```python
from build123d import *

# Parameters (mm, degrees)
SKETCH1_W           = 36
SKETCH1_H           = 36
SKETCH1_W_2         = 30
SKETCH1_H_2         = 30
BOSS_EXTRUDE1_DEPTH = 40
SKETCH2_W           = 30
SKETCH2_H           = 30
BOSS_EXTRUDE2_DEPTH = 3
FILLET_1_R          = 2
FILLET_2_R          = 2
FILLET_3_R          = 1


with BuildPart() as part:
    # Sketch1 → Boss-Extrude1 (new body)
    with BuildSketch(Plane(origin=(0, 0, 0), x_dir=(1, 0, 0), z_dir=(0, 1, 0))):
        with Locations((18, 18)):
            Rectangle(SKETCH1_W, SKETCH1_H)
        with Locations((18, 18)):
            Rectangle(SKETCH1_W_2, SKETCH1_H_2, mode=Mode.SUBTRACT)
    extrude(amount=BOSS_EXTRUDE1_DEPTH)

    # Sketch2 → Boss-Extrude2 (add)
    with BuildSketch(Plane.XZ):
        with Locations((18, -18)):
            Rectangle(SKETCH2_W, SKETCH2_H)
    extrude(amount=-BOSS_EXTRUDE2_DEPTH)

    # Скругление1
    fillet_1_edges = [part.edges().sort_by_distance(p)[0] for p in [
        (0, 20, -36),
        (36, 20, -36),
        (36, 20, 0),
        (0, 20, 0),
    ]]
    fillet(fillet_1_edges, radius=FILLET_1_R)

    # Скругление2
    fillet_2_edges = [part.edges().sort_by_distance(p)[0] for p in [
        (0, 0, -18),
        (18, 0, -36),
        (36, 0, -18),
        (18, 0, 0),
        (35.414213562, 0, -0.585786438),
        (35.414213562, 0, -35.414213562),
        (0.585786438, 0, -0.585786438),
        (0.585786438, 0, -35.414213562),
    ]]
    fillet(fillet_2_edges, radius=FILLET_2_R)

    # Скругление3
    fillet_3_edges = [part.edges().sort_by_distance(p)[0] for p in [
        (3, 21.5, -33),
        (3, 21.5, -3),
        (33, 21.5, -3),
        (33, 21.5, -33),
        (3, 40, -18),
        (18, 40, -3),
        (33, 40, -18),
        (18, 40, -33),
        (18, 3, -33),
        (3, 3, -18),
        (18, 3, -3),
        (33, 3, -18),
    ]]
    fillet(fillet_3_edges, radius=FILLET_3_R)


solid = part.part
```
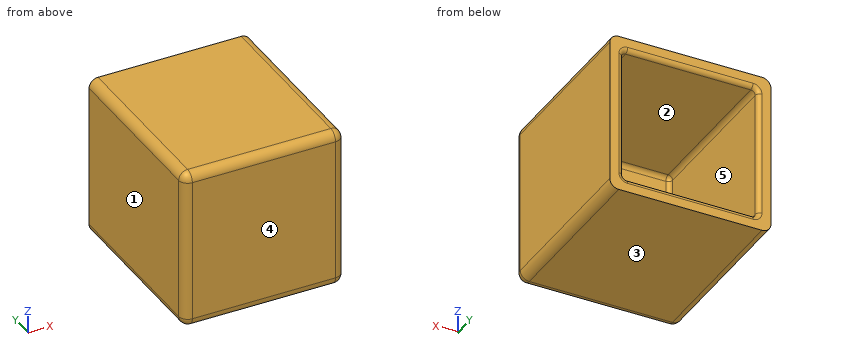
Can you work these out from the model? Positions are in its coordinate system, mm. Face numbers are marked on the shaded views. A direction names the side the tool comes from. Give positions to 0.01 mm unless a question says otherwise; leave off trailing zeros. Order: outer loops, then holes, each group sorted by start corner. A loop starts at its lowest first (then second) coordinate and runs counter-clockwise, first axis right, second up. Notation, with made-up numbers: (17, -17.5) - (31, -17.5) arc R6 ccw to (31, -10.5) - close; hole circle Ø2 at (68.5, -1). An arc over 180 degrees is marked (long way). Use a Markdown table: item, result. Add a question column.
Q1. If we section it at B-B on z = -13.5: Write out the boundary of the cut face in (x, y), plus the area to 3 significant figures.
Q2. On a 3-axis mill with a long thin cutter (end or side, diameter ignored), from which of +Z, -Z, +X, -X, +Y, -Y can I reach the whole of each face in a straight line? I mean the marked faces 4 and 5. Say none if no direction works.
Q3. If we section it at C-C on y = 11: Write out the boundary of the cut face in (x, z), plus the area to 3 significant figures.
Q4. If we section it at A-A on x = 7.5: Write out the boundary of the cut face in (y, z).
Q5. I'm going to push flat-ended pins straight in: pin 1 (8.5 mm diameter, centred on x = 16, z = -14, fed in from +Y); pin 2 (10 mm diameter, centred on x = 22.5, z = -27.5, fed in from +Y). Where does each tip first touch, or does it pass through?
Q6. If we mould it in two halves opening along X, with no side actions, what happens to the marked faces 1, 2 and 3? For each: released by +X, released by -X, zero draft, split by the parting line, or undercut.
Q7. Please list where these lines run through material, in increasing order: line 1 along Z through (x, y) = (24, 34.5); line 2 along X through (y, z) = (36, -31.5); line 3 along Y through (x, z) = (17, -30).
Answers follow:
| question | item | result |
|---|---|---|
| 1 | outline | (0, 2) arc R2 ccw to (2, 0) - (34, 0) arc R2 ccw to (36, 2) - (36, 40) - (34, 40) arc R1 ccw to (33, 39) - (33, 4) arc R1 cw to (32, 3) - (4, 3) arc R1 cw to (3, 4) - (3, 39) arc R1 ccw to (2, 40) - (0, 40) - close |
| 1 | area | 328 mm^2 |
| 2 | face 4 | +Z, -Z, +X, -X, -Y |
| 2 | face 5 | +Y |
| 3 | outline | (0, -34) arc R2 ccw to (2, -36) - (34, -36) arc R2 ccw to (36, -34) - (36, -2) arc R2 ccw to (34, 0) - (2, 0) arc R2 ccw to (0, -2) - close; hole (3, -32) arc R1 ccw to (4, -33) - (32, -33) arc R1 ccw to (33, -32) - (33, -4) arc R1 ccw to (32, -3) - (4, -3) arc R1 ccw to (3, -4) - close |
| 3 | area | 393 mm^2 |
| 4 | outline | (0, -34) arc R2 ccw to (2, -36) - (40, -36) - (40, -34) arc R1 ccw to (39, -33) - (4, -33) arc R1 cw to (3, -32) - (3, -4) arc R1 cw to (4, -3) - (39, -3) arc R1 ccw to (40, -2) - (40, 0) - (2, 0) arc R2 ccw to (0, -2) - close |
| 5 | pin 1 | stops at y = 3 |
| 5 | pin 2 | stops at y = 3.13 |
| 6 | face 1 | released by -X |
| 6 | face 2 | undercut |
| 6 | face 3 | zero draft |
| 7 | line 1 | z = -36 to -33, -3 to 0 |
| 7 | line 2 | x = 0 to 3, 33 to 36 |
| 7 | line 3 | y = 0 to 3 |
